```python
from build123d import *

# Parameters (mm, degrees)
BOSS_EXTRUDE1_DEPTH     = 30
SHELL1_T                = -8
SKETCH3_R               = 3
CUT_EXTRUDE1_DEPTH      = 30
SKETCH4_R               = 3
CUT_EXTRUDE2_DEPTH      = 10
CUT_EXTRUDE3_DEPTH      = 57.107040556
CUT_EXTRUDE3_DEPTH_BACK = 57.107040556
SKETCH8_W               = 3.5
SKETCH8_H               = 8.5


with BuildPart() as part:
    # Sketch2 → Boss-Extrude1 (new body)
    with BuildSketch(Plane(origin=(0, 0, 0), x_dir=(1, 0, 0), z_dir=(0, 1, 0))):
        Polygon((10, -30), (42, -17.5), (42, 0), (0, 0), (0, -30), align=None)
    extrude(amount=BOSS_EXTRUDE1_DEPTH)

    # Shell1
    shell1_openings = [part.faces().sort_by_distance(p)[0] for p in [
        (42, 15, 8.75),
        (26, 15, 23.75),
        (5, 15, 30),
    ]]
    offset(amount=SHELL1_T, openings=shell1_openings, kind=Kind.INTERSECTION)

    # Sketch3 → Cut-Extrude1 (cut)
    with BuildSketch(Plane(origin=(8, 0, 0), x_dir=(0, 0, -1), z_dir=(1, 0, 0))):
        with Locations((-22.5, 15)):
            Circle(SKETCH3_R)
        with Locations((-7.5, 15)):
            Circle(SKETCH3_R)
    extrude(amount=-CUT_EXTRUDE1_DEPTH, mode=Mode.SUBTRACT)

    # Sketch4 → Cut-Extrude2 (cut)
    with BuildSketch(Plane.XY.offset(8)):
        with Locations((16, 15)):
            Circle(SKETCH4_R)
        with Locations((34, 15)):
            Circle(SKETCH4_R)
    extrude(amount=-CUT_EXTRUDE2_DEPTH, mode=Mode.SUBTRACT)

    # Sketch8 → Cut-Extrude3 (cut, two sides: drawn at the far end of the back side and taken through both)
    with BuildSketch(Plane.XY.offset(8).offset(-CUT_EXTRUDE3_DEPTH_BACK)):
        with Locations((7.75, 15)):
            Rectangle(SKETCH8_W, SKETCH8_H)
    extrude(amount=CUT_EXTRUDE3_DEPTH + CUT_EXTRUDE3_DEPTH_BACK, mode=Mode.SUBTRACT)


solid = part.part
```
Verification items for the finished model (mm, model axes). A direction names the side the tool comes from. Coordinates: 2 decimals unless noted, no trailing zeros. Loops run counter-clockwise (first coordinate to the right, second up) from the corner with the lowest first, then second, coordinate; pieces in that order, holes last. Notation, with made-up numbers: (26.25, 67) -> (39.25, 67) arc R29 cw to (39.25, 100) -> close; hole circle Ø10 at (77.25, 11). An arc over 180 degrees is marked (long way). Put each result on its own line as item: value.
1. Thickness scan on line 1 (Y direction, x = 40, z = 12); line 2 (Y direction, x = 16, z = 2.5); line 3 (Z direction, x = 22, y = 11.5). Record the ranges inside material, lowest first.
Result set:
line 1: y = 0 to 8, 22 to 30
line 2: y = 0 to 12, 18 to 30
line 3: z = 0 to 8
2. Tool access check on faces 4 (the face through (21, 22, 16)), 5 (the face through (21, 15, 0)), 6 (the face through (4, 15, 30)), 7 (the face through (7, 10.75, 11)), 8 (the face through (3.042, 12.338, 6.116)). Record the directions out of +Z, -Z, +X, -X, +Y, -Y that give a thin tool (end or side, any length) a straight path to the whole face; none if there is none.
Result set:
face 4: +Z, +X
face 5: -Z, +X, -X, +Y, -Y
face 6: +Z, +X, -X, +Y, -Y
face 7: +Z, -Z
face 8: -X
3. Mould release check, pull along X, two halves, no side actions. Record for faces 1 (the face through (9.5, 15, 4)), 2 (the face through (42, 15, 7)), 3 (the face through (21, 8, 16)): pulls with the +X half, pulls with the -X half, needs draft (parallel to the pull), parting line crosses it, or undercut.
Result set:
face 1: undercut
face 2: pulls with the +X half
face 3: needs draft
4. Section check B-B, the plane y = 15. Record the boundary of the cut face in (x, z).
Result set:
outline: (0, 0) -> (6, 0) -> (6, 4.5) -> (0, 4.5) -> close; (0, 10.5) -> (6, 10.5) -> (6, 19.5) -> (0, 19.5) -> close; (0, 25.5) -> (6, 25.5) -> (6, 30) -> (0, 30) -> close; (9.5, 0) -> (13, 0) -> (13, 8) -> (9.5, 8) -> close; (19, 0) -> (31, 0) -> (31, 8) -> (19, 8) -> close; (37, 0) -> (42, 0) -> (42, 8) -> (37, 8) -> close
5. Gauge pin test, flat ends, axial feed: P1, Ø6, axis at x = 22.5, y = 8, coming from the +Z side; P2, Ø8, axis at x = 16, y = 10, coming from the +Z side; P3, Ø7, axis at x = 29, y = 12, coming from the +Z side; P4, Ø5.5, axis at x = 16, y = 15, coming from the -Z side. Record the tip position at first contact, or that the pin passes through.
Result set:
P1: stops at z = 26.29
P2: stops at z = 29.01
P3: stops at z = 8
P4: passes through
6. Section check D-D, the plane z = 7.5. Record the boundary of the cut face in (x, y), then the cut area to 3 significant figures.
Result set:
outline: (0, 0) -> (42, 0) -> (42, 30) -> (0, 30) -> (0, 18) -> (6, 18) -> (6, 19.25) -> (9.5, 19.25) -> (9.5, 10.75) -> (6, 10.75) -> (6, 12) -> (0, 12) -> close; hole circle Ø6 at (16, 15); hole circle Ø6 at (34, 15)
area: 1,140 mm^2
7. Section check A-A, the plane z = 22.5. Record the boundary of the cut face in (x, y).
Result set:
outline: (0, 0) -> (29.2, 0) -> (29.2, 8) -> (8, 8) -> (8, 10.75) -> (6, 10.75) -> (6, 12) -> (0, 12) -> close; (0, 18) -> (6, 18) -> (6, 19.25) -> (8, 19.25) -> (8, 22) -> (29.2, 22) -> (29.2, 30) -> (0, 30) -> close
8. Section check C-C, the plane x = 15. Record the boundary of the cut face in (y, z), then the cut area to 3 significant figures.
Result set:
outline: (0, 0) -> (12.17, 0) -> (12.17, 8) -> (8, 8) -> (8, 28.05) -> (0, 28.05) -> close; (17.83, 0) -> (30, 0) -> (30, 28.05) -> (22, 28.05) -> (22, 8) -> (17.83, 8) -> close
area: 515 mm^2
